from build123d import *

# Parameters (mm, degrees)
F1_DEPTH     = 18.3
F2_W         = 17.3
F2_H         = 6.1
F3_DEPTH     = 25
F4_R         = 9.6568542495
F5_R         = 5.7941125497
F6_W         = 15
F6_H         = 6.1
F7_DEPTH     = 25
F8_R         = 3
F9_R         = 2
F11_DEPTH    = 7.6
F12_W        = 3.9829482868
F12_H        = 6.1
F13_DEPTH    = 25
F14_T1_DEPTH = 2
F15_DEPTH    = 1
F16_DEPTH    = 1
F17_DEPTH    = 2
F18_DEPTH    = 2
F19_DEPTH    = 0.5
F20_DEPTH    = 0.5


# Not quite as in the source:
# - a fillet or chamfer that OpenCascade refuses, or shapes differently, is made with other operations: its cross-section is extruded or revolved along the edge and cut away or added


with BuildPart() as f1:
    # F0 (on Top) → F1 (new body)
    with BuildSketch(Plane.XY):
        Polygon((4.2331174448, -18.8899510824), (-35.7668825552, -18.8899510824), (-35.7668825552, -20.8899510824), (6.2331174448, -20.8899510824), (6.2331174448, 13.1100489176), (4.2331174448, 13.1100489176), align=None)
    extrude(amount=F1_DEPTH)

    # F2 (on face) → F3 (cut)
    with BuildSketch(Plane(origin=(0, -18.8899510824, 0), x_dir=(-1, 0, 0), z_dir=(0, 1, 0))):
        with Locations((27.1168825552, 9.15)):
            Rectangle(F2_W, F2_H)
    extrude(amount=-F3_DEPTH, mode=Mode.SUBTRACT)

    # F4
    f4_edges = [f1.edges().sort_by_distance(p)[0] for p in [
        (4.233117, -18.889951, 9.15),
    ]]
    fillet(f4_edges, radius=F4_R)

    # F5
    f5_edges = [f1.edges().sort_by_distance(p)[0] for p in [
        (6.233117, -20.889951, 9.15),
    ]]
    fillet(f5_edges, radius=F5_R)

    # F6 (on face) → F7 (cut)
    with BuildSketch(Plane(origin=(4.2331174448, 0, 0), x_dir=(0, -1, 0), z_dir=(-1, 0, 0))):
        with Locations((-5.6100489176, 9.15)):
            Rectangle(F6_W, F6_H)
    extrude(amount=-F7_DEPTH, mode=Mode.SUBTRACT)

    # F8
    f8_edges = [f1.edges().sort_by_distance(p)[0] for p in [
        (5.233117, -1.889951, 6.1),
        (5.233117, -1.889951, 12.2),
    ]]
    fillet(f8_edges, radius=F8_R)

    # F9
    f9_edges = [f1.edges().sort_by_distance(p)[0] for p in [
        (5.233117, 13.110049, 0),
        (5.233117, 13.110049, 18.3),
        (-35.766883, -19.889951, 0),
        (-35.766883, -19.889951, 18.3),
    ]]
    fillet(f9_edges, radius=F9_R)

    # F10 (on face) → F11 (cut)
    with BuildSketch(Plane.XZ.offset(20.8899510824)):
        Polygon((7.5907320715, 6.1), (7.5907320715, 9.2), (7.5907320715, 12.2), (-4.1556255892, 12.2), (-4.1556255892, 6.1), align=None)
    extrude(amount=-F11_DEPTH, mode=Mode.SUBTRACT)

    # F12 (on face) → F13 (cut)
    with BuildSketch(Plane(origin=(0, -18.8899510824, 0), x_dir=(-1, 0, 0), z_dir=(0, 1, 0))):
        with Locations((16.4754084118, 9.15)):
            Rectangle(F12_W, F12_H)
    extrude(amount=-F13_DEPTH, mode=Mode.SUBTRACT)

    # F14: fillet of radius 3.0660512242 on 2 edges, made by hand

    # F14_s2 → F14_t1 (join)
    with BuildSketch(Plane.XZ.offset(18.8899510824)):
        with BuildLine():
            ThreePointArc((-14.4839342684, 9.1660512242), (-15.3819598805, 6.9980256121), (-17.5499854926, 6.1))
            Line((-17.5499854926, 6.1), (-14.4839342684, 6.1))
            Line((-14.4839342684, 6.1), (-14.4839342684, 9.1660512242))
        make_face()
        with BuildLine():
            ThreePointArc((-17.5499854926, 12.2), (-15.3819598805, 11.3019743879), (-14.4839342684, 9.1339487758))
            Line((-14.4839342684, 9.1339487758), (-14.4839342684, 12.2))
            Line((-14.4839342684, 12.2), (-17.5499854926, 12.2))
        make_face()
    extrude(amount=F14_T1_DEPTH)

    # F15 (cut): faces of the model
    f15_faces = [f1.faces().sort_by_distance(p)[0] for p in [
        (1.8734055755, -17.7191060476, 6.1),
        (1.8734055755, -17.7191060476, 12.2),
    ]]
    extrude(f15_faces, amount=-F15_DEPTH, dir=(0, 0, 1), mode=Mode.SUBTRACT)

    # F16 (cut): a face of the model
    f16_faces = [f1.faces().sort_by_distance(p)[0] for p in [
        (1.8734055755, -17.7191060476, 12.2),
    ]]
    extrude(f16_faces, amount=-F16_DEPTH, mode=Mode.SUBTRACT)

    # F17 (cut): a face of the model
    f17_faces = [f1.faces().sort_by_distance(p)[0] for p in [
        (-4.1556255892, -19.8481388351, 9.15),
    ]]
    extrude(f17_faces, amount=-F17_DEPTH, mode=Mode.SUBTRACT)

    # F18 (cut): a face of the model
    f18_faces = [f1.faces().sort_by_distance(p)[0] for p in [
        (4.7863785676, -13.2899510824, 9.15),
    ]]
    extrude(f18_faces, amount=-F18_DEPTH, mode=Mode.SUBTRACT)

    # F19 (cut): a face of the model
    f19_faces = [f1.faces().sort_by_distance(p)[0] for p in [
        (1.6308493787, -17.3698716383, 13.2),
    ]]
    extrude(f19_faces, amount=-F19_DEPTH, mode=Mode.SUBTRACT)

    # F20 (cut): a face of the model
    f20_faces = [f1.faces().sort_by_distance(p)[0] for p in [
        (1.6308493787, -17.3698716383, 5.1),
    ]]
    extrude(f20_faces, amount=-F20_DEPTH, mode=Mode.SUBTRACT)


solid = f1.part
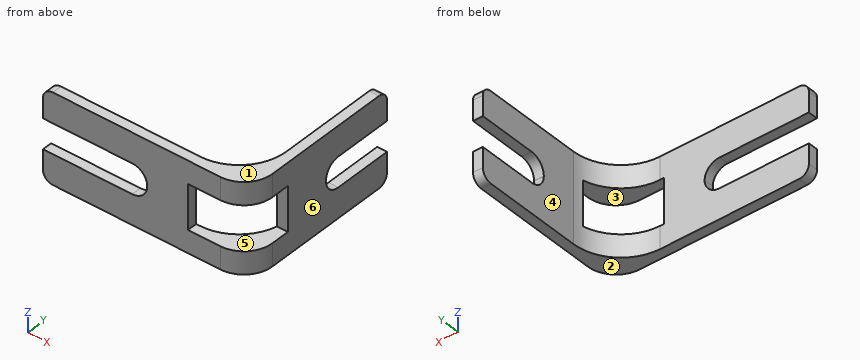
Verification items for the finished model (mm, model axes). Face numbers are marked on the shaded views. A direction names the side the tool comes from. Coordinates: 2 decimals unless noted, no trailing zeros. Write each loop counter-clockwise with the first axis right and the second up, starting at its lowest first coordinate (ties: lowest second). Pieces come first, ordered by that corner, then holes. Notation, with made-up numbers: (1, 54.5) -> (28, 54.5) arc R27 ccw to (28, 89.5) -> close; hole circle Ø8 at (35, 20.25). An arc over 180 degrees is marked (long way). One line per item, written item: value. Start each with the question number.
Q1. Cross-section at D-D on z = 3.25. Enter the section's corners in (x, y).
Q2. Cross-section at A-A on x = -26.5. Enter the section's corners in (y, z), and give its area (3 significant figures).
Q3. Mould release check, pull along Z, two halves, no side actions. Record for the marked faces 1, 2 and 3: pulls with the +Z half, pulls with the -Z half, needs draft (parallel to the pull), parting line crosses it, or undercut.
Q4. Go/stop test with flat-tipped pins: P1, Ø6, axis at y = 5.5, z = 5, coming from the -X side; P2, Ø1.5, axis at x = -31, z = 8.5, coming from the +Y side; P3, Ø2, axis at y = -20.5, z = 10, coming from the +X side; P4, Ø0.7, axis at x = 5.5, z = 8.5, coming from the -Y side. Record where each tip stops, or that it passes through.
Q5. Thickness scan on L1, parallel to X at y = 3, z = 17; L2, parallel to Y at x = -33, z = 13; L3, parallel to X at y = -19, z = 2. Record the ranges inside material, lowest first. Write a range as from..to.
Q6. Access from +Z, -Z, +X, -X, +Y, -Y to the whole of each face (thin tool, end or side, straight path). Record for the marked faces 4, 5 and 6.
Q7. Cross-section at C-C on z = 11. Enter the section's corners in (x, y), and give its area (3 significant figures).
Q8. Cross-section at B-B on y = 3.5. Enter the section's corners in (x, z), and give its area (3 significant figures).
Checked values:
1. outline: (-35.77, -20.89) -> (0.44, -20.89) arc R5.79 ccw to (6.23, -15.1) -> (6.23, 13.11) -> (4.23, 13.11) -> (4.23, -9.23) arc R9.66 cw to (-5.42, -18.89) -> (-35.77, -18.89) -> close
2. outline: (-20.89, 0) -> (-18.89, 0) -> (-18.89, 6.1) -> (-20.89, 6.1) -> close; (-20.89, 12.2) -> (-18.89, 12.2) -> (-18.89, 18.3) -> (-20.89, 18.3) -> close
2. area: 24.4 mm²
3. face 1: pulls with the +Z half
3. face 2: pulls with the -Z half
3. face 3: undercut
4. P1: stops at x = 4.23
4. P2: passes through
4. P3: stops at x = -6.16
4. P4: stops at y = -11.29
5. L1: x = 4.23..6.23
5. L2: y = -20.89..-18.89
5. L3: x = -35.77..4.72
6. face 4: +Z, -Z, -X, +Y
6. face 5: +X, -Y
6. face 6: +Z, -Z, +X, +Y, -Y
7. outline: (-15.12, -20.89) -> (-6.16, -20.89) -> (-6.16, -18.89) -> (-15.12, -18.89) -> close; (4.01, -11.29) -> (6.23, -11.29) -> (6.23, -1.29) -> (4.23, -1.29) -> (4.23, -9.23) arc R9.66 cw to start
7. area: 38.1 mm²
8. outline: (4.23, 0) -> (6.23, 0) -> (6.23, 6.1) -> (4.23, 6.1) -> close; (4.23, 12.2) -> (6.23, 12.2) -> (6.23, 18.3) -> (4.23, 18.3) -> close
8. area: 24.4 mm²
